Design review of the part built by this model. Coordinates are the model's own, in mm. A direction names the side the tool comes from. Give positions to 0.01 mm unless a question says otherwise; leave off trailing zeros. Loops run counter-clockwise (first coordinate to the right, second up) from the corner with the lowest first, then second, coordinate; pieces in that order, holes last. Notation, with made-up numbers: M 35,-36 L 79,-36 A20 cw 79,0 Z; hole C -32,85 d3. An arc over 180 degrees is marked long. Answer as CSV lines item,"result".
```python
from build123d import *

# Parameters (mm, degrees)
F0_R     = 72.7
F0_R_2   = 53.3
F1_DEPTH = 20
F2_T     = -0.7
F3_R     = 1.5


with BuildPart() as f1:
    # F0 (on Top) → F1 (new body)
    with BuildSketch(Plane.XY):
        Circle(F0_R)
        Circle(F0_R_2, mode=Mode.SUBTRACT)
    extrude(amount=F1_DEPTH)

    # F2
    f2_openings = [f1.faces().sort_by_distance(p)[0] for p in [
        (-70.643733, 0, 20),
    ]]
    offset(amount=F2_T, openings=f2_openings)

    # F3
    f3_edges = [f1.edges().sort_by_distance(p)[0] for p in [
        (-72, 0, 0.7),
        (-54, 0, 0.7),
    ]]
    fillet(f3_edges, radius=F3_R)


solid = f1.part
```
1. For faces 1 (the cylindrical face through (-11.706, -52.716, 10.975)), 2 (the flat face through (40, -36, 20)), list the 3-axis set-ups (+Z, -Z, +X, -X, +Y, -Y) from which the entire face can be reached by the end or side of a thin tool; tool diameter is ignored.
Answer block:
face 1,"+Z"
face 2,"+Z, +X, -X, +Y, -Y"
2. For P1, Ø6, axis at y = 57, z = 5.5, coming from the -X side; P2, Ø1, axis at y = -10, z = 16, coming from the +X side; P3, Ø12, axis at x = -37, z = 3.5, coming from the +Y side, all flat-tipped, find the tip position at first contact; note any pin that passes through.
Answer block:
P1,"x = -48.68"
P2,"x = 72.08"
P3,"y = 65.76"
3. To check wall thickness, follow L1, parallel to Y at x = 0, z = 12; L2, parallel to X at y = -22, z = 9.75; L3, parallel to X at y = -26, z = 13.25. State the ranges of each line that lie inside material, in increasing order. Write a range as [from, to].
Answer block:
L1,"[-72.7, -72], [-54, -53.3], [53.3, 54], [72, 72.7]"
L2,"[-69.29, -68.56], [-49.32, -48.55], [48.55, 49.32], [68.56, 69.29]"
L3,"[-67.89, -67.14], [-47.33, -46.53], [46.53, 47.33], [67.14, 67.89]"
4. We need section A-A, the plane x = 0. Write out the cut boundary in (y, z).
Answer block:
outline,"M -72.7,0 L -53.3,0 L -53.3,20 L -54,20 L -54,2.2 A1.5 cw -55.5,0.7 L -70.5,0.7 A1.5 cw -72,2.2 L -72,20 L -72.7,20 Z; M 53.3,0 L 72.7,0 L 72.7,20 L 72,20 L 72,2.2 A1.5 cw 70.5,0.7 L 55.5,0.7 A1.5 cw 54,2.2 L 54,20 L 53.3,20 Z"
5. We need section B-B, the plane z = 13.25. Write out the cut boundary in (x, y).
Answer block:
outline,"C 0,0 d145.4; C 0,0 d108; hole C 0,0 d144; hole C 0,0 d106.6"
